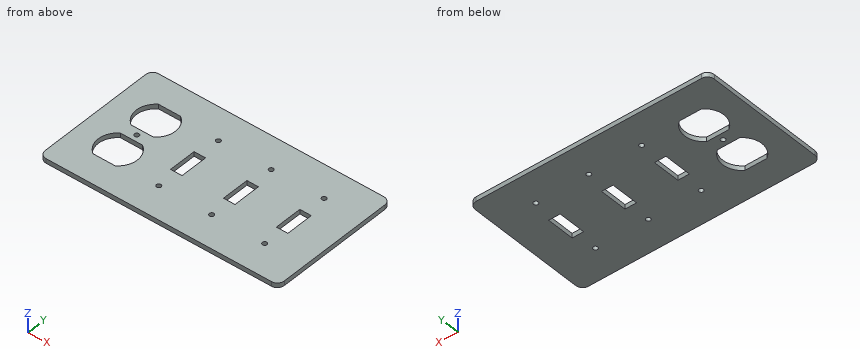
from build123d import *

# Parameters (mm, degrees)
F0_W     = 208
F0_H     = 115
F0_R     = 2
F0_W_2   = 10
F0_H_2   = 24
F1_DEPTH = 4
F2_R     = 6
F4_R     = 2
F4_R_2   = 17
F5_DEPTH = 25
F6_W     = 27.550638
F6_H     = 3.205147
F6_W_2   = 29.028984
F6_H_2   = 3.037915
F6_W_3   = 33.224199
F6_H_3   = 3
F7_DEPTH = 4


with BuildPart() as f1:
    # F0 (on Top) → F1 (new body)
    with BuildSketch(Plane.XY):
        with Locations((104, 57.5)):
            Rectangle(F0_W, F0_H)
        with Locations((81, 27)):
            Circle(F0_R, mode=Mode.SUBTRACT)
        with Locations((81, 57)):
            Rectangle(F0_W_2, F0_H_2, mode=Mode.SUBTRACT)
        with Locations((127, 27)):
            Circle(F0_R, mode=Mode.SUBTRACT)
        with Locations((173, 27)):
            Circle(F0_R, mode=Mode.SUBTRACT)
        with Locations((127, 57)):
            Rectangle(F0_W_2, F0_H_2, mode=Mode.SUBTRACT)
        with Locations((173, 57)):
            Rectangle(F0_W_2, F0_H_2, mode=Mode.SUBTRACT)
        with Locations((81, 88)):
            Circle(F0_R, mode=Mode.SUBTRACT)
        with Locations((127, 88)):
            Circle(F0_R, mode=Mode.SUBTRACT)
        with Locations((173, 88)):
            Circle(F0_R, mode=Mode.SUBTRACT)
    extrude(amount=F1_DEPTH)

    # F2
    f2_edges = [f1.edges().sort_by_distance(p)[0] for p in [
        (0, 115, 2),
        (208, 115, 2),
        (208, 0, 2),
        (0, 0, 2),
    ]]
    fillet(f2_edges, radius=F2_R)

    # F4 (on Top) → F5 (cut)
    with BuildSketch(Plane.XY):
        with Locations((36, 57.5)):
            Circle(F4_R)
        with Locations((36, 77)):
            Circle(F4_R_2)
        with Locations((36, 38)):
            Circle(F4_R_2)
    extrude(amount=F5_DEPTH, mode=Mode.SUBTRACT)

    # F6 (on face) → F7 (join)
    with BuildSketch(Plane.XY.offset(4)):
        Polygon((32.74464, 94.836249), (25.32669, 91), (46.063566, 91), (43.255925, 94.420469), align=None)
        with Locations((37.412647, 61.397426)):
            Rectangle(F6_W, F6_H)
        with Locations((37.197317, 53.518957)):
            Rectangle(F6_W_2, F6_H_2)
        with Locations((36.739217, 22.5)):
            Rectangle(F6_W_3, F6_H_3)
    extrude(amount=-F7_DEPTH)


solid = f1.part
Source: CAD feature listing. Evaluate the final solid. Frame: model axes, mm. Give positions to 0.01 mm unless a question says otherwise; leave off trailing zeros. Write each loop counter-clockwise with the first axis right and the second up, starting at its lowest first coordinate (ties: lowest second). Pieces come first, ordered by that corner, then holes. Notation, with made-up numbers: M 81.25,-1.5 L 108.25,-1.5 A19 ccw 108.25,17.5 Z; hole C -39.5,68.25 d5. An arc over 180 degrees is marked long. Return JSON: item names as keys, results as strings. Group by question number.
1) Pin query (flat end, axial travel): P1, Ø5, axis at x = 81, y = 27, coming from the -Z side. Return the tip coordinate at first contact, or that it passes through.
2) Material intervals for line 1 along Y through (x, z) = (173, 2.1); line 2 along X through (y, z) = (61.5, 2.1); line 3 along X through (y, z) = (57.5, 1.95), sorted ascending. Write a range as [from, to].
3) Cut plane B-B, the plane y = 43. Output: boundary loops of the cut face in (x, z).
4) Cut plane D-D, the plane z = 2.1. Give the number of separate pieces and of enclosed holes in the cut face, plus the area to 3 significant figures.
5) Cut plane C-C, the plane x = 173. Output: boundary loops of the cut face in (y, z), plus the area to 3 significant figures.
6) Cut plane A-A, the plane x = 36. Output: boundary loops of the cut face in (y, z).
Recorded:
{
 "1": {"P1": "stops at z = 0"},
 "2": {"line 1": "y = [0, 25], [29, 45], [69, 86], [90, 115]", "line 2": "x = [0, 76], [86, 122], [132, 168], [178, 208]", "line 3": "x = [0, 34], [38, 76], [86, 122], [132, 168], [178, 208]"},
 "3": {"outline": "M 0,0 L 19.75,0 L 19.75,4 L 0,4 Z; M 52.25,0 L 208,0 L 208,4 L 52.25,4 Z"},
 "4": {"separate pieces": "1", "enclosed holes": "12", "area": "21,400 mm²"},
 "5": {"outline": "M 0,0 L 25,0 L 25,4 L 0,4 Z; M 29,0 L 45,0 L 45,4 L 29,4 Z; M 69,0 L 86,0 L 86,4 L 69,4 Z; M 90,0 L 115,0 L 115,4 L 90,4 Z", "area": "332 mm²"},
 "6": {"outline": "M 0,0 L 24,0 L 24,4 L 0,4 Z; M 52,0 L 55.5,0 L 55.5,4 L 52,4 Z; M 59.5,0 L 63,0 L 63,4 L 59.5,4 Z; M 91,0 L 115,0 L 115,4 L 91,4 Z"}
}
